Autodesk Inventor part; units mm, degrees
sketch "Sketch1" plane through (0, 0, 0) normal (0, 0, 1) x (1, 0, 0)
  line L0 (-43.75, -9) -> (43.75, -9)
  line L1 (43.75, -9) -> (43.75, 9)
  line L2 (43.75, 9) -> (-43.75, 9)
  line L3 (-43.75, 9) -> (-43.75, -9)
  line L4 (-43.75, -9) -> (43.75, 9) construction
  line L5 (43.75, -9) -> (-43.75, 9) construction
  point P0 (0, 0)
  dimension "d0" = 87.5
  dimension "d1" = 18
extrude "Extrusion1" add sketch "Sketch1" along normal mid plane 15
sketch "Sketch3" plane through (-43.75, 9, 7.5) normal (0, 1, 0) x (1, 0, 0)
  line L0 (0, 15) -> (87.5, 0.25)
  line L1 (87.5, 15) -> (87.5, 0) construction
  line L2 (87.5, 0.25) -> (87.5, 15)
  line L3 (87.5, 15) -> (0, 15)
  point P0 (43.75, 7.5)
  point P1 (87.5, 7.625)
  dimension "d5" = 0.25
extrude "Extrusion2" cut sketch "Sketch3" along normal through all both and the other way through all
sketch "Sketch5" plane through (-43.75, -9, 7.5) normal (-1, 0, 0) x (0, 0, 1)
  line L0 (-3.95, 2.75) -> (-10.3, 2.75)
  line L1 (-10.3, 2.75) -> (-10.3, 15.25)
  line L2 (-10.3, 15.25) -> (-3.95, 15.25)
  line L3 (-3.95, 15.25) -> (-3.95, 2.75)
  line L4 (-3.95, 2.75) -> (-10.3, 15.25) construction
  line L5 (-10.3, 2.75) -> (-3.95, 15.25) construction
  line L6 (0, 18) -> (0, 0) construction
  line L7 (-15, 0) -> (-15, 18) construction
  point P0 (-7.5, 9)
  point P1 (-7.125, 9)
  dimension "d14" = 12.5
  dimension "d28" = 3.95
  dimension "d29" = 4.7
extrude "Extrusion4" add sketch "Sketch5" along normal blind 38.75
sketch "Sketch7" plane through (0, 0, -2.8) normal (0, 0, 1) x (1, 0, 0)
  line L0 (-82.5, 6.25) -> (-82.5, -6.25) construction
  circle A0 centre (-131.7, 0) radius 49
  line L1 (43.75, -9) -> (43.75, 9)
  line L2 (-82.5, -6.25) -> (-83.1002, -6.25)
  line L3 (-82.5, 6.25) -> (-83.1002, 6.25)
  line L4 (-82.5, -6.25) -> (-82.5, 6.25)
  point P0 (0, 0)
  point P1 (43.75, 0)
  point P2 (-82.5, 0)
  dimension "d23" = 98
  dimension "d24" = 175.45
extrude "Extrusion5" add sketch "Sketch7" along normal blind 5.65 contours A0 L3 L4 L2
fillet "Fillet2" radius 5 2 edges at (0, 9, -0.125) (0, -9, -0.125)
equation "\"d25\" = d15"
properties part number "BracoRobotico_0003_002" material "Rubber"
Input: part model. Units: mm. Frame: model coordinates. A direction names the side the tool comes from. Round coordinates to 2 decimals unless told otherwise and drop trailing zeros. Write each loop counter-clockwise with the first axis right and the second up, starting at its lowest first coordinate (ties: lowest second). Pieces come first, ordered by that corner, then holes.
1) Cut plane B-B (x = -64.5). Return the cut outline in (y, z).
2) Ray query, L1, parallel to Z at x = -76.5, y = -1.25; L2, parallel to Y at x = -42, z = -2.5; L3, parallel to Y at x = -54, z = -1.5. Return the intervals inside material, ascending.
3) Contact query for flat-ended pins moving along their axis: P1, Ø8, axis at x = 6, z = -1, coming from the +Y side; P2, Ø3, axis at x = -55, z = 0.5, coming from the -Y side; P3, Ø1.9, axis at x = -55.5, z = 1, coming from the +Y side. Output: stop coordinate, or through.
4) Draft query along Y for faces 5 (the flat face through (-0.612, 0.056, -0.228)), 6 (the cylindrical face through (-82.7, 0.1, 0)), 7 (the flat face through (-21, -9, 5)), 8 (the flat face through (-63, 6.25, 0)). Return one class per face: pulls with the +Y half, pulls with the -Y half, needs draft (parallel to the pull), parting line crosses it, or undercut.
5) Cut plane A-A (y = -1). Return the cut outline in (x, z).
6) Reachability of faces 1 (the flat face through (-63, -6.25, 0)), 2 (the flat face through (-63, 0, 3.55)), 3 (the cylindrical face through (0.38, -7.57, 1.46)), 4 (the flat face through (-64, 0, -2.8)) from +Z, -Z, +X, -X, +Y, -Y: full face, straight path, thin tool, end or side. Return the list, or none.
Geometry says:
1. outline: (-6.25, -2.8) - (6.25, -2.8) - (6.25, 3.55) - (-6.25, 3.55) - close
2. L1: z = -2.8 to 3.55
2. L2: y = -8.99 to 8.99
2. L3: y = -6.25 to 6.25
3. P1: stops at y = 8.1
3. P2: stops at y = -6.25
3. P3: stops at y = 6.25
4. face 5: needs draft
4. face 6: undercut
4. face 7: pulls with the -Y half
4. face 8: pulls with the +Y half
5. outline: (-82.71, -2.8) - (-43.75, -2.8) - (-43.75, -7.5) - (43.75, 7.25) - (43.75, 7.5) - (-43.75, 7.5) - (-43.75, 3.55) - (-82.5, 3.55) - (-82.5, 2.85) - (-82.71, 2.85) - close
6. face 1: +Z, -Z, -X, -Y
6. face 2: +Z, -X, +Y, -Y
6. face 3: -Z, +X, -Y
6. face 4: -Z, -X, +Y, -Y
